```python
from build123d import *

# Parameters (mm, degrees)
F0_W     = 660
F0_H     = 300
F0_R     = 75.5
F0_R_2   = 90.5
F0_R_3   = 41
F0_R_4   = 50
F1_DEPTH = 75
F2_DEPTH = 32


with BuildPart() as f1:
    # F0 (on Top) → F1 (new body)
    with BuildSketch(Plane.XY):
        Rectangle(F0_W, F0_H)
        with Locations((-220, 0)):
            Circle(F0_R, mode=Mode.SUBTRACT)
        Circle(F0_R_2, mode=Mode.SUBTRACT)
        with Locations((220, 0)):
            Circle(F0_R, mode=Mode.SUBTRACT)
        with Locations((-220, 0)):
            Circle(F0_R)
        with Locations((-220, 0)):
            Circle(F0_R_3, mode=Mode.SUBTRACT)
        Circle(F0_R_2)
        Circle(F0_R_4, mode=Mode.SUBTRACT)
        with Locations((220, 0)):
            Circle(F0_R)
        with Locations((220, 0)):
            Circle(F0_R_3, mode=Mode.SUBTRACT)
    extrude(amount=F1_DEPTH)

    # F0 (on Top) → F2 (cut)
    with BuildSketch(Plane.XY):
        with Locations((-220, 0)):
            Circle(F0_R)
        with Locations((-220, 0)):
            Circle(F0_R_3, mode=Mode.SUBTRACT)
        Circle(F0_R_2)
        Circle(F0_R_4, mode=Mode.SUBTRACT)
        with Locations((220, 0)):
            Circle(F0_R)
        with Locations((220, 0)):
            Circle(F0_R_3, mode=Mode.SUBTRACT)
    extrude(amount=F2_DEPTH, mode=Mode.SUBTRACT)


solid = f1.part
```
Work out the finished part from the listing and answer in its coordinate system (mm). A direction names the side the tool comes from. Give positions to 0.01 mm unless a question says otherwise; leave off trailing zeros. Order: outer loops, then holes, each group sorted by start corner. A loop starts at its lowest first (then second) coordinate and runs counter-clockwise, first axis right, second up. Notation, with made-up numbers: M 64.25,11.5 L 96.25,11.5 A23 cw 96.25,45.5 Z; hole C 22.5,74.25 d1. An arc over 180 degrees is marked long. Return JSON: item names as keys, results as strings.
1) Section B-B, the plane z = 46 is taken. Write down the section's boundary in (x, y).
Resolved:
{"outline": "M -330,-150 L 330,-150 L 330,150 L -330,150 Z; hole C -220,0 d82; hole C 0,0 d100; hole C 220,0 d82"}
2) Straight lines are drawn through the part: line 1 along Y through (x, z) = (0, 62); line 2 along Y through (x, z) = (220, 7); line 3 along X through (y, z) = (-35.5, 38.5). For each, find the intervals that lie inside material, in ascending order. Write a range as [from, to].
Resolved:
{"line 1": "[-150, -50], [50, 150]", "line 2": "[-150, -75.5], [75.5, 150]", "line 3": "[-330, -240.51], [-199.49, -35.21], [35.21, 199.49], [240.51, 330]"}
3) For a pull along Y with two mould halves and no side action, classify faces 1 (the flat face through (39, -39, 32)), 2 (the flat face through (330, -2, 37)), 3 (the flat face through (-5, -150, 37)) as +Y half, -Y half, draft (parallel to the pull), parting line (faces both ways), or undercut.
Resolved:
{"face 1": "undercut", "face 2": "draft", "face 3": "-Y half"}
4) A tool of negligible diameter and unlimited length cuts with its end or side. For faces 4 (the flat face through (-78, 69, 0)), 5 (the cylindrical face through (86.32, 27.18, 15.78)), from which of +Z, -Z, +X, -X, +Y, -Y can it reach the whole face along a straight path? Write none if from no direction.
Resolved:
{"face 4": "-Z, +X, -X, +Y, -Y", "face 5": "-Z"}
5) Section C-C, the plane x = 0 is taken. Write down the section's boundary in (y, z).
Resolved:
{"outline": "M -150,0 L -90.5,0 L -90.5,32 L -50,32 L -50,75 L -150,75 Z; M 50,32 L 90.5,32 L 90.5,0 L 150,0 L 150,75 L 50,75 Z"}
6) Section A-A, the plane y = 0 is taken. Write down the section's boundary in (x, z).
Resolved:
{"outline": "M -330,0 L -295.5,0 L -295.5,32 L -261,32 L -261,75 L -330,75 Z; M -179,32 L -144.5,32 L -144.5,0 L -90.5,0 L -90.5,32 L -50,32 L -50,75 L -179,75 Z; M 50,32 L 90.5,32 L 90.5,0 L 144.5,0 L 144.5,32 L 179,32 L 179,75 L 50,75 Z; M 261,32 L 295.5,32 L 295.5,0 L 330,0 L 330,75 L 261,75 Z"}
7) Section D-D, the plane z = 16 is taken. Write down the section's boundary in (x, y), plus the area to 3 significant figures.
Resolved:
{"outline": "M -330,-150 L 330,-150 L 330,150 L -330,150 Z; hole C -220,0 d151; hole C 0,0 d181; hole C 220,0 d151", "area": "136,000 mm^2"}
